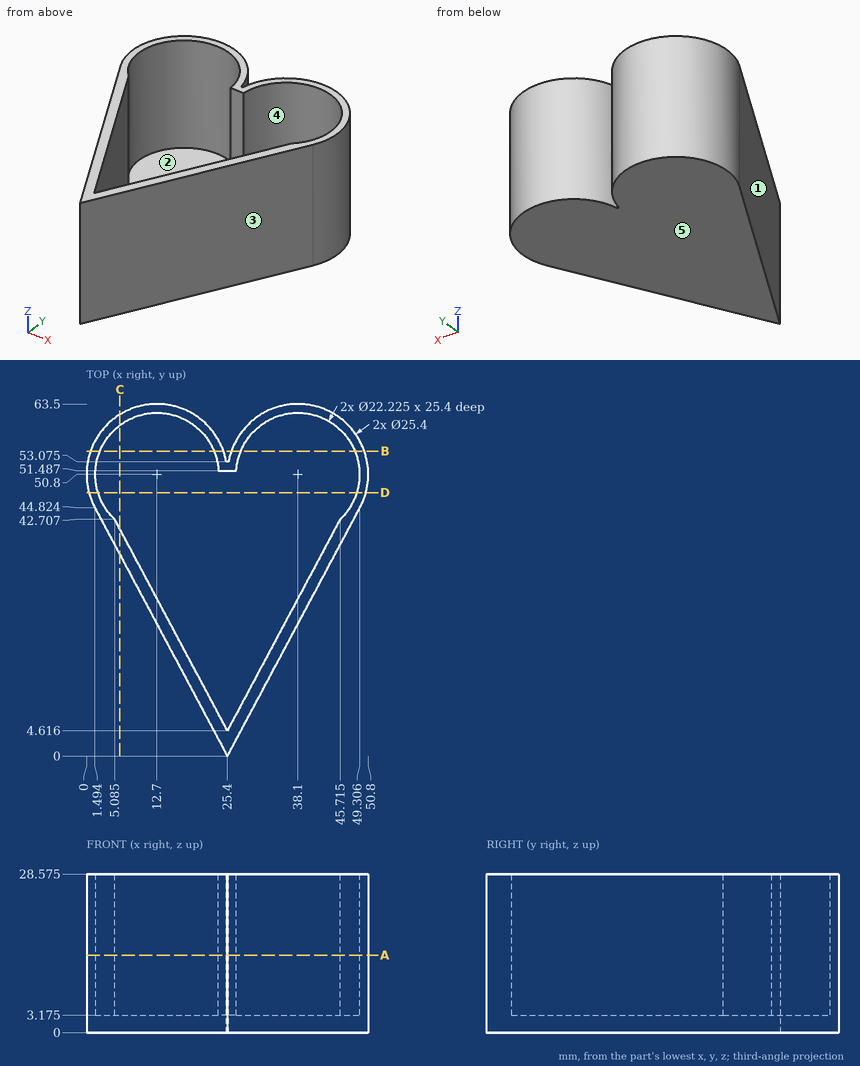
Geometry: see drawing. Coordinates: mm, zero at the bounding-box minimum. A direction names the side the tool comes from. Coordinates: 2 decimals unless noted, no trailing zeros. Write each loop counter-clockwise with the first axis right and the second up, starting at its lowest first coordinate (ties: lowest second). Pieces come first, ordered by that corner, then holes.
1) Section A-A on z = 14. Output: boundary loops of the cut face in (x, y) (1 decimal).
2) Set-up query: the marked faces 1 and 2. Return all of +Z, -Z, +X, -X, +Y, -Y with unobstructed straight access to the full face (end or side cutting, diameter ignored); none if empty.
3) Material intervals for line 1 along X through (y, z) = (50.8, 14.25); line 2 along X through (y, z) = (58, 12) (1 decimal); line 3 along X through (y, z) = (52, 11.5), sorted ascending.
4) Section B-B on y = 55. Output: boundary loops of the cut face in (x, z) (1 decimal).
5) Mould query, pull axis X, two halves, no side actions, for the marked faces 3, 4 and 5. Classes: pulls with the +X half, pulls with the -X half, needs draft (parallel to the pull), parting line crosses it, or undercut.
6) Section C-C on x = 6. Output: boundary loops of the cut face in (y, z) (1 decimal), and give its area (3 significant figures).
7) Pin query (flat end, axial travel): pin 1 Ø6 at (y, z) = (13.5, 7) entering from -X; pin 2 Ø2.5 at (x, z) = (25.5, 18.5) entering from -Y; pin 3 Ø2 at (y, z) = (15, 4) entering from +X. Return the tip coordinate at first contact, or that it passes through.
8) Section D-D on y = 47.5. Output: boundary loops of the cut face in (x, z) (1 decimal).
Check result:
1. outline: (1.5, 44.8) - (25.4, 0) - (49.3, 44.8) arc R12.7 ccw (long way) to (25.6, 53.1) - (25.2, 53.1) arc R12.7 ccw (long way) to start; hole (5.1, 42.7) - (25.4, 4.6) - (45.7, 42.7) arc R11.1 ccw (long way) to (27, 51.5) - (23.8, 51.5) arc R11.1 ccw (long way) to start
2. face 1: +Z, -Z, -X, -Y
2. face 2: +Z
3. line 1: x = 0 to 1.59, 49.21 to 50.8
3. line 2: x = 2.2 to 4.2, 21.2 to 23.2, 27.6 to 29.6, 46.6 to 48.6
3. line 3: x = 0.06 to 1.65, 23.75 to 27.05, 49.15 to 50.74
4. outline: (0.7, 0) - (24.7, 0) - (24.7, 28.6) - (23, 28.6) - (23, 3.2) - (2.4, 3.2) - (2.4, 28.6) - (0.7, 28.6) - close; (26.1, 0) - (50.1, 0) - (50.1, 28.6) - (48.4, 28.6) - (48.4, 3.2) - (27.8, 3.2) - (27.8, 28.6) - (26.1, 28.6) - close
5. face 3: pulls with the +X half
5. face 4: undercut
5. face 5: needs draft
6. outline: (36.4, 0) - (61.6, 0) - (61.6, 28.6) - (59.7, 28.6) - (59.7, 3.2) - (41, 3.2) - (41, 28.6) - (36.4, 28.6) - close
6. area: 246 mm2
7. pin 1: stops at x = 16.6
7. pin 2: stops at y = 0
7. pin 3: stops at x = 33.93
8. outline: (0.4, 0) - (50.4, 0) - (50.4, 28.6) - (48.7, 28.6) - (48.7, 3.2) - (2.1, 3.2) - (2.1, 28.6) - (0.4, 28.6) - close
